```python
from build123d import *

# Parameters (mm, degrees)
F2_R     = 20
F3_R     = 5
F5_DEPTH = 1
F6_DEPTH = 1
F7_COUNT = 4


with BuildPart() as f1:
    # F0 (on Front) → F1 (revolve)
    with BuildSketch(Plane.XZ):
        Polygon((0, 27.0555268526), (0, 29.0555268526), (-1.1768030475, 27.9391527077), (-5.1872356048, 10.792308032), (-2.8048087843, -60.7303120611), (-2.8048087843, -70.9474980831), (-1.6, -70.9444731474), (-1.6, -61.4324361086), (-4, 10.6177468147), align=None)
    revolve(axis=Axis((0, 0, 28.0555268526), (0, 0, -1)))

    # F2
    f2_edges = [f1.edges().sort_by_distance(p)[0] for p in [
        (5.187236, 0, 10.792308),
    ]]
    fillet(f2_edges, radius=F2_R)

    # F3
    f3_edges = [f1.edges().sort_by_distance(p)[0] for p in [
        (1.176803, 0, 27.939153),
    ]]
    fillet(f3_edges, radius=F3_R)

    # F4 (on Front) → F5 (join)
    with BuildSketch(Plane.XZ):
        Polygon((-2.6657825802, -70.9118023515), (-2.6657825802, -60.9118023515), (-16.3306742907, -70.9118023515), align=None)
    extrude(amount=F5_DEPTH)



with BuildPart() as f6:
    # F4 (on Front) → F6 (new body)
    with BuildSketch(Plane.XZ):
        Polygon((-2.6657825802, -70.9118023515), (-2.6657825802, -60.9118023515), (-16.3306742907, -70.9118023515), align=None)
    extrude(amount=-F6_DEPTH)


with BuildPart() as f1_1:
    add(f1.part)

    add(f6.part)  # F7 merges F6
    # F7: F1, F6 ×4 about axis
    f7_axis = Axis((0, 0, -65.9047495574), (0, 0, -1))
    for i in range(1, F7_COUNT):
        add(f1.part.rotate(f7_axis, i * 360 / F7_COUNT))
        add(f6.part.rotate(f7_axis, i * 360 / F7_COUNT))


solid = f1_1.part
```
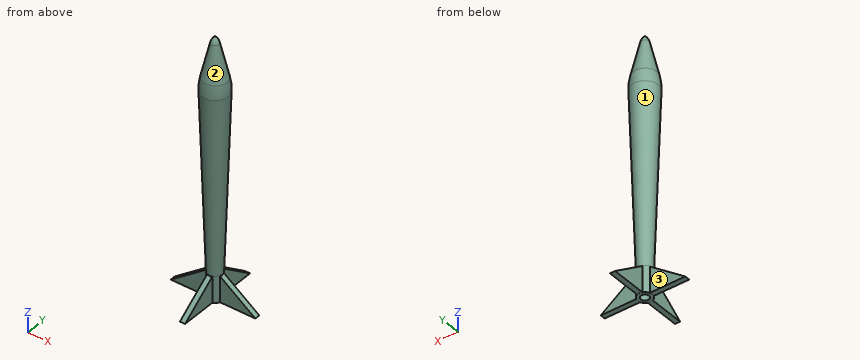
For this review, take the finished solid that the model builds, in its own axes (mm). Face numbers are marked on the shaded views. Round coordinates to 2 decimals unless told otherwise and drop trailing zeros. Write each loop counter-clockwise with the first axis right and the second up, starting at its lowest first coordinate (ties: lowest second). Pieces come first, ordered by that corner, then holes. Notation, with made-up numbers: (32, 53.25) - (71, 53.25) arc R21 ccw to (71, 59.25) - close; hole circle Ø1 at (-8, -34). An arc over 180 degrees is marked (long way). Use CSV: the item, a comma, the result in double quotes.
1) Add section A-A on z = -50.5. Write out the cut boundary in (x, y), and give its area (3 significant figures).
Conclusion:
outline,"circle Ø6.29 at (0, 0); hole circle Ø3.93 at (0, 0)"
area,"19.0 mm^2"
2) Add section C-C on x = 7.5. Write out the cut boundary in (y, z), and give its area (3 significant figures).
Conclusion:
outline,"(-1, -70.91) - (1, -70.91) - (1, -64.45) - (-1, -64.45) - close"
area,"12.9 mm^2"
3) Clearance check with flat-ended pins moving along their axes: pin 1 Ø11 at (x, z) = (9, -65) entering from -Y; pin 2 Ø10 at (y, z) = (-3, 7) entering from -X; pin 3 Ø1.5 at (x, y) = (1.5, -6.5) entering from -Z; pin 4 Ø10 at (y, z) = (10, -57.5) entering from +X. State where each tip first meets the part, or that it passes through.
Conclusion:
pin 1,"stops at y = -1"
pin 2,"stops at x = -5.11"
pin 3,"stops at z = -70.91"
pin 4,"passes through"
4) Wall thickness on line 1 along Y through (x, z) = (0, -64.5); line 2 along X through (y, z) = (-2, -34.5); line 3 along X through (y, z) = (0, -64): over which ranges is each line inside the solid? List them lowest first. Write a range as from..to.
Conclusion:
line 1,"y = -7.57..-1.6, 1.6..7.57"
line 2,"x = -3.09..-1.5, 1.5..3.09"
line 3,"x = -6.89..-1.6, 1.6..6.89"
5) Add section B-B on y = -12. Write out the cut boundary in (x, z).
Conclusion:
outline,"(-1, -70.91) - (1, -70.91) - (1, -67.74) - (-1, -67.74) - close"
6) The part is to be moulded in two halves that separate along Z. For the marked faces 1, 2 and 3, say which applies: pulls with the +Z half, pulls with the -Z half, needs draft (parallel to the pull), parting line crosses it, or undercut.
Conclusion:
face 1,"undercut"
face 2,"pulls with the +Z half"
face 3,"needs draft"
7) Add section D-D on z = 3. Write out the cut boundary in (x, y), and give its area (3 significant figures).
Conclusion:
outline,"circle Ø9.86 at (0, 0); hole circle Ø7.49 at (0, 0)"
area,"32.2 mm^2"
